```python
from build123d import *

# Parameters (mm, degrees)
SKETCH1_W           = 17.84
SKETCH1_H           = 19.05
BOSS_EXTRUDE1_DEPTH = 0.79
SKETCH2_R           = 0.795
SKETCH2_W           = 0.789999944
SKETCH2_H           = 4.76
CUT_EXTRUDE1_DEPTH  = 2.54
SKETCH4_R           = 0.32
CUT_EXTRUDE2_DEPTH  = 27.111150875
FILLET1_R           = 1.590000122


with BuildPart() as part:
    # Sketch1 → Boss-Extrude1 (new body)
    with BuildSketch(Plane(origin=(0, 0, 0), x_dir=(1, 0, 0), z_dir=(0, 1, 0))):
        with Locations((8.92, 9.525)):
            Rectangle(SKETCH1_W, SKETCH1_H)
    extrude(amount=BOSS_EXTRUDE1_DEPTH)

    # Sketch2 → Cut-Extrude1 (cut)
    with BuildSketch(Plane(origin=(0, 0.79, 0), x_dir=(1, 0, 0), z_dir=(0, 1, 0))):
        with Locations(Location((12.76, 2.54, 0), (0, 0, 270))):
            Circle(SKETCH2_R)
        with Locations(Location((3.81, 2.54, 0), (0, 0, 270))):
            Circle(SKETCH2_R)
        with Locations(Location((3.81, 9.53, 0), (0, 0, 270))):
            Circle(SKETCH2_R)
        with Locations(Location((12.76, 9.53, 0), (0, 0, 270))):
            Circle(SKETCH2_R)
        with Locations(Location((12.76, 16.51, 0), (0, 0, 270))):
            Circle(SKETCH2_R)
        with Locations(Location((3.81, 16.51, 0), (0, 0, 270))):
            Circle(SKETCH2_R)
        with Locations((17.445000028, 11.91)):
            Rectangle(SKETCH2_W, SKETCH2_H)
        with Locations((17.445000028, 2.38)):
            Rectangle(SKETCH2_W, SKETCH2_H)
    extrude(amount=-CUT_EXTRUDE1_DEPTH, mode=Mode.SUBTRACT)

    # Sketch4 → Cut-Extrude2 (cut, through all)
    with BuildSketch(Plane.XY):
        with Locations((17.445000028, 0.395)):
            Circle(SKETCH4_R)
        with BuildLine():
            Line((17.84, 0.79), (17.445000028, 0.79))
            ThreePointArc((17.445000028, 0.79), (17.724307207, 0.674307179), (17.840000028, 0.395))
            Line((17.84, 0.395), (17.84, 0.79))
        make_face()
        with BuildLine():
            ThreePointArc((17.840000028, 0.395), (17.724307207, 0.115692821), (17.445000028, 0))
            Line((17.445000028, 0), (17.84, 0))
            Line((17.84, 0), (17.84, 0.395))
        make_face()
    extrude(amount=-CUT_EXTRUDE2_DEPTH, mode=Mode.SUBTRACT)

    # Fillet1
    fillet1_edges = [part.edges().sort_by_distance(p)[0] for p in [
        (0, 0.395, -19.05),
        (0, 0.395, 0),
    ]]
    fillet(fillet1_edges, radius=FILLET1_R)


solid = part.part
```
Work out the finished part from the listing and answer in its coordinate system (mm). Give positions to 0.01 mm unless a question says otherwise; leave off trailing zeros. Loops run counter-clockwise (first coordinate to the right, second up) from the corner with the lowest first, then second, coordinate; pieces in that order, holes last. Notation, with made-up numbers: M 89.25,28 L 109.25,28 A24 ccw 109.25,57 Z; hole C 4,-9 d9. An arc over 180 degrees is marked long. One line per item, written item: value. Start each with the question number.
1. Find section C-C (z = -16.51). Give the vertices of the cut face in (x, y) (3 decimals), and give its area (3 significant figures).
2. Determine the mould class of faces 1 (the face through (12.276, 0.401, -10.161)), 2 (the face through (3.105, 0.401, -2.173)), 3 (the face through (0.45, 0.4, -18.57)), 4 (the face through (9, 0, -10)) for opening direction Z: released by +Z, released by -Z, zero draft, split by the parting line, or undercut.
3. Find section A-A (z = -2.54). Give the vertices of the cut face in (x, y) (3 decimals).
4. Find the intervals of material crossed by probe 1 along X at (y, z) = (0.7, -2.75); probe 2 along X at (y, z) = (0.3, -11), in increasing order.
5. Find section D-D (y = 0.25). State how many separate pieces and enclosed holes the cut face has, and give its area (3 significant figures).
6. Find section B-B (x = 12.76). Give the vertices of the cut face in (y, z) (3 decimals).
Reported:
1. outline: M 0,0 L 3.015,0 L 3.015,0.79 L 0,0.79 Z; M 4.605,0 L 11.965,0 L 11.965,0.79 L 4.605,0.79 Z; M 13.555,0 L 17.445,0 A0.395 ccw 17.445,0.79 L 13.555,0.79 Z; hole C 17.445,0.395 d0.64
1. area: 11.2 mm²
2. face 1: undercut
2. face 2: undercut
2. face 3: released by -Z
2. face 4: zero draft
3. outline: M 0,0 L 3.015,0 L 3.015,0.79 L 0,0.79 Z; M 4.605,0 L 11.965,0 L 11.965,0.79 L 4.605,0.79 Z; M 13.555,0 L 17.05,0 L 17.05,0.79 L 13.555,0.79 Z
4. probe 1: x = 0 to 3.04, 4.58 to 11.99, 13.53 to 17.05
4. probe 2: x = 0 to 17.05
5. separate pieces: 3
5. enclosed holes: 6
5. area: 314 mm²
6. outline: M 0,-19.05 L 0.79,-19.05 L 0.79,-17.305 L 0,-17.305 Z; M 0,-15.715 L 0.79,-15.715 L 0.79,-10.325 L 0,-10.325 Z; M 0,-8.735 L 0.79,-8.735 L 0.79,-3.335 L 0,-3.335 Z; M 0,-1.745 L 0.79,-1.745 L 0.79,0 L 0,0 Z
